Input: part model. Units: mm. Frame: model coordinates. Face numbers are marked on the shaded views. A direction names the side the tool comes from. Round coordinates to 2 decimals unless told otherwise and drop trailing zeros. Loops run counter-clockwise (first coordinate to the right, second up) from the corner with the lowest first, then second, coordinate; pieces in that order, holes last. Notation, with made-up numbers: (58, -14) -> (88, -14) arc R21 ccw to (88, -2) -> close; hole circle Ø1 at (-16, -33.75). An arc over 180 degrees is marked (long way). Answer as a JSON object with one key per item and string values. Group by question number.
Item 1: Set-up query: the marked faces 4, 5 and 6. Return all of +Z, -Z, +X, -X, +Y, -Y with unobstructed straight access to the full face (end or side cutting, diameter ignored); none if empty.
Item 2: Draft query along X for the marked faces 1, 2 and 3. Return one class per face: released by +X, released by -X, zero draft, split by the parting line, or undercut.
Item 3: Section query B-B on x = 0. Return loops of the section in (y, z).
Item 4: Section query D-D on y = -19.5. Return loops of the section in (x, z).
Item 5: Material intervals for line 1 (Y direction, x = 0, z = 3.8); line 2 (X direction, y = -26, z = 3.2); line 3 (Y direction, x = 1, z = 3.2), sorted ascending. Write a range as [from, to].
Item 6: Section query A-A on y = 0. Return loops of the section in (x, z).
Item 7: Pin query (flat end, axial travel): pin 1 (1.6 mm diameter, centred on y = 11, z = 2, fed in from -X); pin 2 (1.5 mm diameter, centred on y = 11, z = 3, fed in from +X); pin 3 (1.5 mm diameter, centred on y = -15.5, z = 3.5, fed in from -X). Return the tip coordinate at first contact, or that it passes through.
Item 8: Section query C-C on z = 2.3. Return loops of the section in (x, y).
from build123d import *

# Parameters (mm, degrees)
SKETCH2_R           = 1.5
BOSS_EXTRUDE1_DEPTH = 5


with BuildPart() as part:
    # Sketch2 → Boss-Extrude1 (new body)
    with BuildSketch(Plane.XY):
        with BuildLine():
            Line((5, -8.660254038), (5, -33))
            ThreePointArc((5, -33), (0, -38), (-5, -33))
            Line((-5, -33), (-5, -8.542766751))
            ThreePointArc((-5, -8.542766751), (-5.270994803, -8.136429895), (-5.750270597, -8.230464661))
            Line((-5.750270597, -8.230464661), (-7.072992385, -9.544016527))
            ThreePointArc((-7.072992385, -9.544016527), (-9.548009447, -9.543873182), (-9.547579415, -7.068856154))
            Line((-9.547579415, -7.068856154), (-7.570062095, -5.051082723))
            ThreePointArc((-7.570062095, -5.051082723), (-6.875312951, -3.018601992), (-8.606609983, -1.747277927))
            Line((-8.606609983, -1.747277927), (-11.749999685, -1.747277927))
            ThreePointArc((-11.749999685, -1.747277927), (-13.499796954, 0.002924757), (-11.74959427, 1.752722026))
            Line((-11.74959427, 1.752722026), (-8.924497087, 1.781187396))
            ThreePointArc((-8.924497087, 1.781187396), (-6.996054349, 2.727106472), (-7.321304353, 4.850280211))
            Line((-7.321304353, 4.850280211), (-9.544016527, 7.072992385))
            ThreePointArc((-9.544016527, 7.072992385), (-9.543729855, 9.547866086), (-7.068856154, 9.547579415))
            Line((-7.068856154, 9.547579415), (-5.051082723, 7.570062095))
            ThreePointArc((-5.051082723, 7.570062095), (-3.018601992, 6.875312951), (-1.747277927, 8.606609983))
            Line((-1.747277927, 8.606609983), (-1.747277927, 11.749999685))
            ThreePointArc((-1.747277927, 11.749999685), (0.002924781, 13.499999673), (1.752722026, 11.74959427))
            Line((1.752722026, 11.74959427), (1.752722026, 9.845200125))
            ThreePointArc((1.752722026, 9.845200125), (9.849506187, 1.728359878), (5, -8.660254038))
        make_face()
        with Locations((0, -33)):
            Circle(SKETCH2_R, mode=Mode.SUBTRACT)
        Circle(SKETCH2_R, mode=Mode.SUBTRACT)
    extrude(amount=BOSS_EXTRUDE1_DEPTH)


solid = part.part
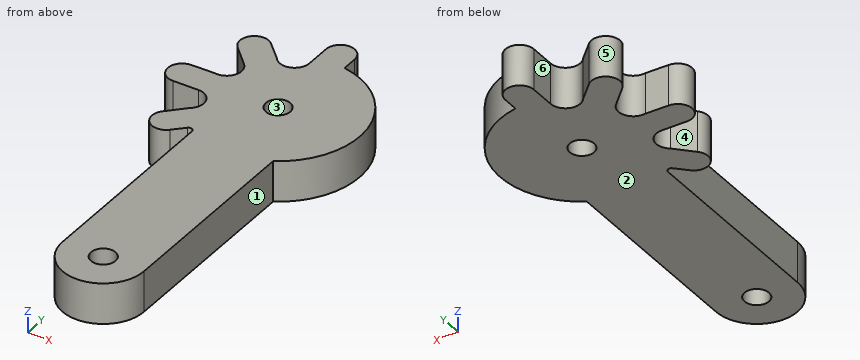
Solved:
{
 "1": {"face 4": "+Z, -Z, -X", "face 5": "+Z, -Z", "face 6": "+Z, -Z, +Y"},
 "2": {"face 1": "released by +X", "face 2": "zero draft", "face 3": "undercut"},
 "3": {"outline": "(-38, 0) -> (-34.5, 0) -> (-34.5, 5) -> (-38, 5) -> close; (-31.5, 0) -> (-1.5, 0) -> (-1.5, 5) -> (-31.5, 5) -> close; (1.5, 0) -> (13.5, 0) -> (13.5, 5) -> (1.5, 5) -> close"},
 "4": {"outline": "(-5, 0) -> (5, 0) -> (5, 5) -> (-5, 5) -> close"},
 "5": {"line 1": "[-38, -34.5], [-31.5, -1.5], [1.5, 13.5]", "line 2": "[-5, 5]", "line 3": "[-37.9, -34.12], [-31.88, -1.12], [1.12, 13.19]"},
 "6": {"outline": "(-13.5, 0) -> (-1.5, 0) -> (-1.5, 5) -> (-13.5, 5) -> close; (1.5, 0) -> (10, 0) -> (10, 5) -> (1.5, 5) -> close"},
 "7": {"pin 1": "x = -1.75", "pin 2": "x = 1.75", "pin 3": "x = -5"},
 "8": {"outline": "(-11.75, -1.75) -> (-8.61, -1.75) arc R1.81 cw to (-7.57, -5.05) -> (-9.55, -7.07) arc R1.75 ccw to (-7.07, -9.54) -> (-5.75, -8.23) arc R0.44 cw to (-5, -8.54) -> (-5, -33) arc R5 ccw to (5, -33) -> (5, -8.66) arc R10 ccw to (1.75, 9.85) -> (1.75, 11.75) arc R1.75 ccw to (-1.75, 11.75) -> (-1.75, 8.61) arc R1.81 cw to (-5.05, 7.57) -> (-7.07, 9.55) arc R1.75 ccw to (-9.54, 7.07) -> (-7.32, 4.85) arc R1.81 cw to (-8.92, 1.78) -> (-11.75, 1.75) arc R1.75 ccw to start; hole circle Ø3 at (0, -33); hole circle Ø3 at (0, 0)"}
}
